from build123d import *

# Parameters (mm, degrees)
BOSS_EXTRUDE1_DEPTH = 18
SHELL1_START        = 2
SHELL1_DEPTH        = 14
CUT_EXTRUDE1_REACH  = 1157.717
SKETCH2_R           = 1.5


# Read off the part's stored shape, not the designer's step: Shell1
with BuildPart() as part:
    # Sketch1 → Boss-Extrude1 (new body)
    with BuildSketch(Plane.XY):
        with BuildLine():
            Line((0, 0), (1125, 0))
            ThreePointArc((1125, 0), (1154.992825207, 30.656076303), (1123.688161208, 59.971304259))
            Line((1123.688161208, 59.971304259), (770, 44.490434753))
            Line((770, 44.490434753), (760, 44.490434753))
            Line((760, 44.490434753), (750, 39.5))
            Line((750, 39.5), (750, 34.5))
            Line((750, 34.5), (770.437279597, 34.5))
            Line((770.437279597, 34.5), (1124.125440805, 49.980869506))
            ThreePointArc((1124.125440805, 49.980869506), (1144.995216805, 30.437384202), (1125, 10))
            Line((1125, 10), (0, 10))
            Line((0, 10), (0, 0))
        make_face()
    extrude(amount=BOSS_EXTRUDE1_DEPTH)

    # Shell1 outline → Shell1 (cut)
    with BuildSketch(Plane.XY.offset(SHELL1_START)):
        with BuildLine():
            Line((815.73732715, 44.490434753), (760, 44.490434753))
            Line((760, 44.490434753), (750, 39.5))
            Line((750, 39.5), (750, 36.5))
            Line((750, 36.5), (770.393530714, 36.5))
            Line((770.393530714, 36.5), (1124.037984886, 51.978956457))
            ThreePointArc((1124.037984886, 51.978956457), (1146.994738485, 30.481122622), (1125, 8))
            Line((1125, 8), (0, 8))
            Line((0, 8), (0, 2))
            Line((0, 2), (1125, 2))
            ThreePointArc((1125, 2), (1152.993303526, 30.612337883), (1123.775617127, 57.973217308))
            Line((1123.775617127, 57.973217308), (815.73732715, 44.490434753))
        make_face()
    extrude(amount=SHELL1_DEPTH, mode=Mode.SUBTRACT)

    # Sketch2 → Cut-Extrude1 (cut, up to next)
    with BuildSketch(Plane(origin=(0, 36.5, 0), x_dir=(1, 0, 0), z_dir=(0, 1, 0)), mode=Mode.PRIVATE) as cut_extrude1_sk1:
        with Locations(Location((754, -9, 0), (0, 0, 180))):
            Circle(SKETCH2_R)
    cut_extrude1_tool1 = extrude(cut_extrude1_sk1.sketch, amount=-CUT_EXTRUDE1_REACH, mode=Mode.PRIVATE) & part.part
    # Sketch2 → Cut-Extrude1 (cut, up to next)
    with BuildSketch(Plane(origin=(0, 36.5, 0), x_dir=(1, 0, 0), z_dir=(0, 1, 0)), mode=Mode.PRIVATE) as cut_extrude1_sk2:
        with Locations(Location((762, -9, 0), (0, 0, 180))):
            Circle(SKETCH2_R)
    cut_extrude1_tool2 = extrude(cut_extrude1_sk2.sketch, amount=-CUT_EXTRUDE1_REACH, mode=Mode.PRIVATE) & part.part
    add(cut_extrude1_tool1.solids().sort_by_distance((754, 36.5, 9))[0], mode=Mode.SUBTRACT)
    add(cut_extrude1_tool2.solids().sort_by_distance((762, 36.5, 9))[0], mode=Mode.SUBTRACT)


solid = part.part
Can you work these out from the model? Positions are in its coordinate system, mm. A direction names the side the tool comes from. Give positions to 0.01 mm unless a question says otherwise; leave off trailing zeros. Order: outer loops, then holes, each group sorted by start corner. A loop starts at its lowest first (then second) coordinate and runs counter-clockwise, first axis right, second up. Notation, with made-up numbers: M 71,20.5 L 75,20.5 A18 cw 75,52.5 Z; hole C 25,20 d10. An arc over 180 degrees is marked long. Use one line per item in the form item = value. Start each with the question number.
Item 1: Will these pins go through, and if not, where does the flat tip stop? pin 1 Ø4 at (x, z) = (662, 7.5) entering from +Y; pin 2 Ø3 at (y, z) = (20.5, 15) entering from -X; pin 3 Ø1 at (y, z) = (49.5, 4) entering from +X; pin 4 Ø5 at (x, y) = (720, 14.5) entering from +Z.
Item 2: We'd pull the mould along Z, two halves only. Please class faces 5 (the flat face through (949.32, 52.34, 8.87)), 6 (the flat face through (660, 8, 18)), 7 (the cylindrical face through (1153, 30, 9)), 8 (the flat face through (660, 8, 0)): +Z half, -Z half, draft (parallel to the pull), parting line (faces both ways), or undercut.
Item 3: If I drill on line 1 along Z through (x, y) = (754, 36); line 2 along Y through (x, z) = (173.5, 7.5); line 3 along Z through (x, y) = (277.5, 7), over which ranges is the centre line in solid material (lowest first)?
Item 4: For faces 1 (the flat face through (570, 10, 9)), 2 (the flat face through (944.806, 42.132, 8.874)), 3 (the cylindrical face through (1146.98, 30.97, 8.9)), 4 (the flat face through (555, 0, 9)), which set-ups out of +Z, -Z, +X, -X, +Y, -Y let a thin tool reach every point of the face, with its end or its side?
Item 5: If we section it at A-A (x = 1039.5): Write out the boundary of the cut face in (y, z).
Outcome:
q1.pin_1 = 10
q1.pin_2 = 1141.7
q1.pin_3 = 1148.22
q1.pin_4 = through
q2.face_5 = draft
q2.face_6 = +Z half
q2.face_7 = undercut
q2.face_8 = -Z half
q3.line_1 = 0 to 7.5, 10.5 to 18
q3.line_2 = 0 to 2, 8 to 10
q3.line_3 = 0 to 2, 16 to 18
q4.face_1 = +Z, -Z, -X
q4.face_2 = +Z, -Z
q4.face_3 = none
q4.face_4 = +Z, -Z, +X, -X, -Y
q5.outline = M 0,0 L 10,0 L 10,18 L 0,18 Z; M 46.28,0 L 56.29,0 L 56.29,18 L 46.28,18 Z; hole M 2,2 L 8,2 L 8,16 L 2,16 Z; hole M 48.28,2 L 54.28,2 L 54.28,16 L 48.28,16 Z
